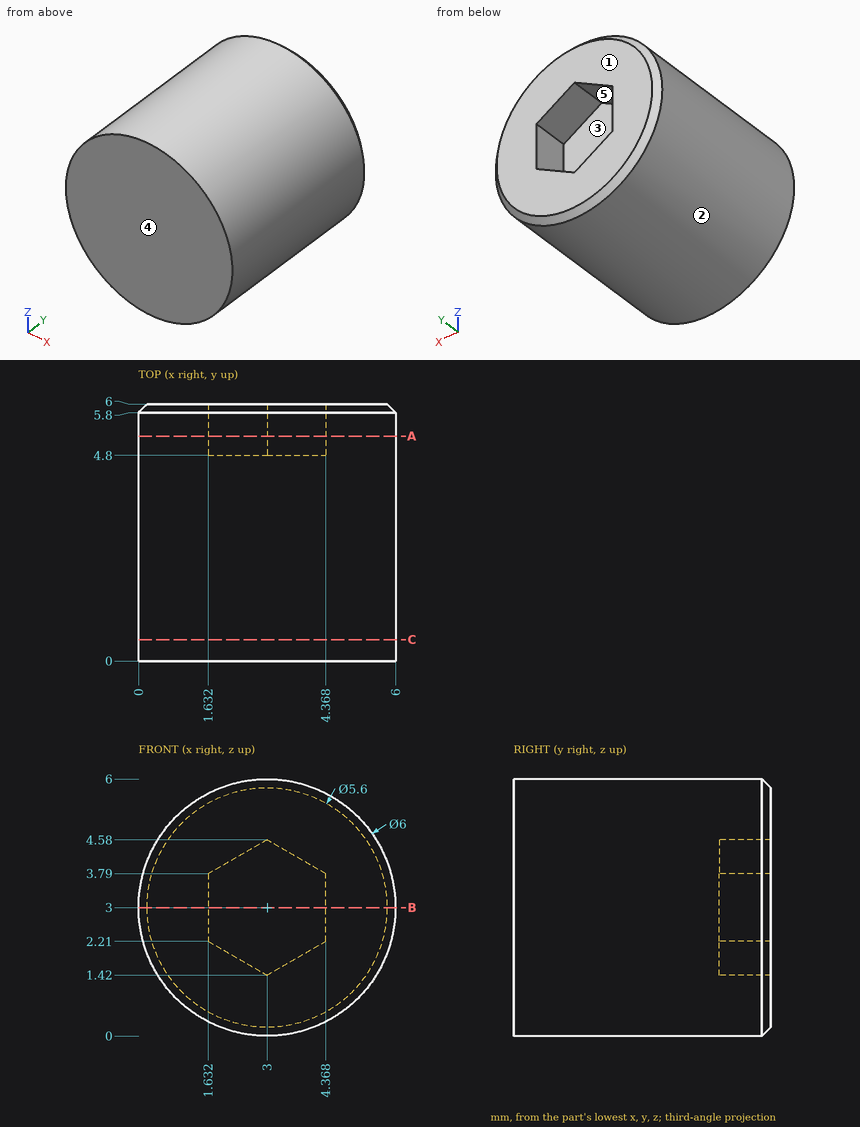
Drawing for the job (mm, zero at the part's lowest x, y, z). A direction names the side the tool comes from. Give positions to 0.01 mm unless a question says otherwise; leave off trailing zeros. Loops run counter-clockwise (first coordinate to the right, second up) from the corner with the lowest first, then second, coordinate; pieces in that order, holes last. Notation, with made-up numbers: (-37, -33.5) - (-24, -33.5) arc R30 cw to (-24, 3.5) - close; hole circle Ø8 at (78.25, 62.25). An arc over 180 degrees is marked (long way). Write item = value, one per line. Start each with the question number.
1) Tool access for the marked faces 4 and 5: list every direction of +Z, -Z, +X, -X, +Y, -Y with a clear straight run to the whole face (end or side of a thin tool).
2) Band-saw the part on A-A on y = 5.25. Give the cut face in (x, z), plus the area to 3 significant figures.
3) Pull direction X, two halves, no side cores. Call the marked faces 1, 2 and 3: +X half, -X half, draft (parallel to the pull), parting line (faces both ways), or undercut.
4) Band-saw the part on C-C on y = 0.5. Give the cut face in (x, z), plus the area to 3 significant figures.
5) Drop flat-ended pins along their axis: pin 1 Ø1.5 at (x, y) = (1.5, 1.5) entering from +Z (1 decimal); pin 2 Ø0.6 at (y, z) = (5.5, 3.5) entering from +X; pin 3 Ø3 at (x, z) = (2, 2.5) entering from +Y. Give the stop position or say it passes through.
6) Band-saw the part on B-B on z = 3. Give the cut face in (x, y).
7) Probe probe 1 along X at (y, z) = (5, 3.05); probe 2 along Y at (x, z) = (2.2, 2.9); probe 3 along X at (y, z) = (5, 1.75) (1 decimal). List the from-to ranges inside material, lowest first. Write a range as from..to.
Final values:
q1.face_4 = +Z, -Z, +X, -X, -Y
q1.face_5 = +Y
q2.outline = circle Ø6 at (3, 3); hole (1.63, 2.21) - (3, 1.42) - (4.37, 2.21) - (4.37, 3.79) - (3, 4.58) - (1.63, 3.79) - close
q2.area = 21.8 mm²
q3.face_1 = draft
q3.face_2 = parting line
q3.face_3 = undercut
q4.outline = circle Ø6 at (3, 3)
q4.area = 28.3 mm²
q5.pin_1 = 5.9
q5.pin_2 = 5.99
q5.pin_3 = 6
q6.outline = (0, 0) - (6, 0) - (6, 5.8) - (5.8, 6) - (4.37, 6) - (4.37, 4.8) - (1.63, 4.8) - (1.63, 6) - (0.2, 6) - (0, 5.8) - close
q7.probe_1 = 0..1.63, 4.37..6
q7.probe_2 = 0..4.8
q7.probe_3 = 0.3..2.4, 3.6..5.7
